from build123d import *

# Parameters (mm, degrees)
CROQUIS1_W              = 2.5
CROQUIS1_H              = 37
SALIENTE_EXTRUIR1_DEPTH = 3
CORTAR_EXTRUIR7_REACH   = 74.534
CROQUIS10_R             = 1
CROQUIS12_R             = 1
CORTAR_EXTRUIR9_DEPTH   = 10


with BuildPart() as part:
    # Croquis1 → Saliente-Extruir1 (new body)
    with BuildSketch(Plane.XY):
        with Locations((-7.257787801, 53.928529755)):
            Rectangle(CROQUIS1_W, CROQUIS1_H)
    extrude(amount=SALIENTE_EXTRUIR1_DEPTH)

    # Croquis10 → Cortar-Extruir7 (cut, up to next)
    with BuildSketch(Plane(origin=(-6.007787801, 0, 0), x_dir=(0, 0, -1), z_dir=(1, 0, 0)), mode=Mode.PRIVATE) as cortar_extruir7_sk1:
        with Locations(Location((-1.5, 70.40205312, 0), (0, 0, 90))):
            Circle(CROQUIS10_R)
    cortar_extruir7_tool1 = extrude(cortar_extruir7_sk1.sketch, amount=-CORTAR_EXTRUIR7_REACH, mode=Mode.PRIVATE) & part.part
    # Croquis10 → Cortar-Extruir7 (cut, up to next)
    with BuildSketch(Plane(origin=(-6.007787801, 0, 0), x_dir=(0, 0, -1), z_dir=(1, 0, 0)), mode=Mode.PRIVATE) as cortar_extruir7_sk2:
        with BuildLine():
            Line((-3, 70.40205312), (-3, 72.428529755))
            Line((-3, 72.428529755), (0, 72.428529755))
            Line((0, 72.428529755), (0, 70.40205312))
            ThreePointArc((0, 70.40205312), (-1.5, 71.90205312), (-3, 70.40205312))
        make_face()
    cortar_extruir7_tool2 = extrude(cortar_extruir7_sk2.sketch, amount=-CORTAR_EXTRUIR7_REACH, mode=Mode.PRIVATE) & part.part
    add(cortar_extruir7_tool1.solids().sort_by_distance((-6.007788, 70.402053, 1.5))[0], mode=Mode.SUBTRACT)
    add(cortar_extruir7_tool2.solids().sort_by_distance((-6.007788, 71.938281, 1.5))[0], mode=Mode.SUBTRACT)

    # Croquis12 → Cortar-Extruir9 (cut)
    with BuildSketch(Plane(origin=(-6.007787801, 0, 0), x_dir=(0, 0, -1), z_dir=(1, 0, 0))):
        with Locations(Location((-1.541120901, 36.722060173, 0), (0, 0, 90))):
            Circle(CROQUIS12_R)
    extrude(amount=-CORTAR_EXTRUIR9_DEPTH, mode=Mode.SUBTRACT)


solid = part.part
Source: CAD feature listing. Evaluate the final solid. Frame: model axes, mm. Give positions to 0.01 mm unless a question says otherwise; leave off trailing zeros. Write each loop counter-clockwise with the first axis right and the second up, starting at its lowest first coordinate (ties: lowest second). Pieces come first, ordered by that corner, then holes. Notation, with made-up numbers: (-5, 46) -> (15, 46) arc R21 ccw to (15, 84) -> close; hole circle Ø7 at (-27.75, 62). An arc over 180 degrees is marked (long way). Return JSON: item names as keys, results as strings. Group by question number.
1. Section B-B, the plane x = -7.6. Output: boundary loops of the cut face in (y, z), then the cut area to 3 significant figures.
2. Section A-A, the plane z = 2.2. Output: boundary loops of the cut face in (x, y).
3. Material intervals for line 1 (Y direction, x = -7.7, z = 1.6); line 2 (Y direction, x = -7.85, z = 1.8); line 3 (Z direction, x = -7.4, y = 69.5), sorted ascending. Write a range as from..to.
4. Mould query, pull axis Y, two halves, no side actions, for faces 1 (the face through (-7.24, 71.9, 1.47)), 2 (the face through (-6.008, 53, 1)), 3 (the face through (-7.24, 71.326, 1.117)). Classes: +Y half, -Y half, draft (parallel to the pull), parting line (faces both ways), or undercut.
Determined:
{
 "1": {"outline": "(35.43, 0) -> (70.4, 0) arc R1.5 ccw to (70.4, 3) -> (35.43, 3) -> close; hole circle Ø2 at (36.72, 1.54); hole circle Ø2 at (70.4, 1.5)", "area": "102 mm2"},
 "2": {"outline": "(-8.51, 35.43) -> (-6.01, 35.43) -> (-6.01, 35.97) -> (-8.51, 35.97) -> close; (-8.51, 37.47) -> (-6.01, 37.47) -> (-6.01, 69.69) -> (-8.51, 69.69) -> close; (-8.51, 71.12) -> (-6.01, 71.12) -> (-6.01, 71.73) -> (-8.51, 71.73) -> close"},
 "3": {"line 1": "y = 35.43..35.72, 37.72..69.41, 71.4..71.9", "line 2": "y = 35.43..35.76, 37.69..69.45, 71.36..71.87", "line 3": "z = 0..1.07, 1.93..3"},
 "4": {"face 1": "+Y half", "face 2": "draft", "face 3": "undercut"}
}
